```python
from build123d import *

# Parameters (mm, degrees)
SKETCH048_W            = 600
SKETCH048_H            = 60
PAD003_DEPTH           = 450
SKETCH049_W            = 612
SKETCH049_H            = 50
PAD010_DEPTH           = 456
SKETCH050_W            = 712
SKETCH050_H            = 1012
PAD011_DEPTH           = 6
CUT001_PLACEMENT_ANGLE = 180


with BuildPart() as body002:
    # Sketch048 → Pad003 (new body, symmetric)
    with BuildSketch(Plane.XZ):
        with Locations((0, 30)):
            Rectangle(SKETCH048_W, SKETCH048_H)
    extrude(amount=PAD003_DEPTH, both=True)


with BuildPart() as cut001:
    # Sketch049 → Pad010 (new body, symmetric)
    with BuildSketch(Plane.XZ):
        with Locations((0, 25)):
            Rectangle(SKETCH049_W, SKETCH049_H)
    extrude(amount=PAD010_DEPTH, both=True)

    # Sketch050 (on Face3 of Pad010) → Pad011 (join)
    with BuildSketch(Plane(origin=(0, 0, 50), x_dir=(-1, 0, 0), z_dir=(0, 0, 1))):
        Rectangle(SKETCH050_W, SKETCH050_H)
    extrude(amount=PAD011_DEPTH)

    # Cut001: cut Body002
    add(body002.part, mode=Mode.SUBTRACT)


with BuildPart() as cut001_1:
    # Cut001 placement: moved
    add(cut001.part.rotate(Axis((0, 0, 0), (0, 1, 0)), CUT001_PLACEMENT_ANGLE))


solid = cut001_1.part
```
Here's how the part is built. I have some questions about the finished solid (model axes, mm). A direction names the side the tool comes from. Give positions to 0.01 mm unless a question says otherwise; leave off trailing zeros. Loops run counter-clockwise (first coordinate to the right, second up) from the corner with the lowest first, then second, coordinate; pieces in that order, holes last. Notation, with made-up numbers: M 23,80.5 L 46,80.5 A24 cw 46,96.5 Z; hole C 46,-14.75 d8. An arc over 180 degrees is marked long. Use one line per item in the form item = value. Start each with the question number.
Q1. Thinking about a two-plate mould opening in X: for faces 4 (the flat face through (4, 450, -28)), 5 (the flat face through (-318, -40, -56)), 6 (the flat face through (306, -6, -25)), which applies, +X half, -X half, draft (parallel to the pull), parting line (faces both ways), or undercut?
Q2. Will these pins go through, and if not, where does the flat tip stop? pin 1 Ø8 at (x, z) = (-55.5, -27.5) entering from -Y; pin 2 Ø3 at (x, z) = (255.5, -7) entering from +Y; pin 3 Ø25 at (y, z) = (-120, -23) entering from -X.
Q3. If we section it at B-B (x = -52): Write out the boundary of the cut face in (y, z).
Q4. Which directions (+Z, -Z, +X, -X, +Y, -Y) give clear straight access to the entire face, cutting with the end or side of a thin tool? Please do faces 1 (the flat face through (4, 456, -25)), 2 (the flat face through (4, -456, -25)), 3 (the flat face through (300, -6, -28)).
Q5. I need wall thicknesses on line 1 along X through (y, z) = (221, -49.5); line 2 along Y through (x, z) = (-264, -8.5); line 3 along Y through (x, z) = (-291.5, -50.5). Which ranges of each line are inside material? Lowest first, please.
Q6. If we section it at C-C (z = -33.5): Write out the boundary of the cut face in (x, y), then the cut area to 3 significant figures.
Q7. If we section it at A-A (y = -309.5): Write out the boundary of the cut face in (x, z), then the cut area to 3 significant figures.
Taken from the geometry:
q1.face_4 = undercut
q1.face_5 = draft
q1.face_6 = +X half
q2.pin_1 = -456
q2.pin_2 = 456
q2.pin_3 = -306
q3.outline = M -506,-56 L -450,-56 L -450,0 L -456,0 L -456,-50 L -506,-50 Z; M 450,-56 L 506,-56 L 506,-50 L 456,-50 L 456,0 L 450,0 Z
q4.face_1 = +Z, +X, -X, +Y
q4.face_2 = +Z, +X, -X, -Y
q4.face_3 = +Z, -Z
q5.line_1 = -306 to -300, 300 to 306
q5.line_2 = -456 to -450, 450 to 456
q5.line_3 = -506 to -450, 450 to 506
q6.outline = M -306,-456 L 306,-456 L 306,456 L -306,456 Z; hole M -300,-450 L 300,-450 L 300,450 L -300,450 Z
q6.area = 18,100 mm^2
q7.outline = M -356,-56 L -300,-56 L -300,0 L -306,0 L -306,-50 L -356,-50 Z; M 300,-56 L 356,-56 L 356,-50 L 306,-50 L 306,0 L 300,0 Z
q7.area = 1,270 mm^2
